CAD build for the part. Positions are in the model's coordinates, mm. A direction names the side the tool comes from. Round coordinates to 2 decimals unless told otherwise and drop trailing zeros. Loops run counter-clockwise (first coordinate to the right, second up) from the corner with the lowest first, then second, coordinate; pieces in that order, holes last. Notation, with made-up numbers: M 32,-32.5 L 50,-32.5 A10 ccw 50,-27.5 Z; hole C 14,71.25 d2. An arc over 180 degrees is marked long. Use one line per item in the form item = value.
Autodesk Inventor part; units mm, degrees
ref_plane "YZ Plane" through (0, 0, 0) normal (1, 0, 0) x (0, 1, 0)
ref_plane "XZ Plane" through (0, 0, 0) normal (0, 1, 0) x (-1, 0, 0)
ref_plane "XY Plane" through (0, 0, 0) normal (0, 0, 1) x (1, 0, 0)
sketch "スケッチ1" plane through (0, 0, 0) normal (0, 0, 1) x (1, 0, 0)
  line L0 (-17.5, 11) -> (17.5, 11)
  line L1 (17.5, 11) -> (17.5, -11)
  line L2 (17.5, -11) -> (-17.5, -11)
  line L3 (-17.5, -11) -> (-17.5, 11)
  point P0 (0, 0)
  point P1 (-17.5, 0)
  point P2 (0, 11)
  dimension "d0" = 35
  dimension "d1" = 22
extrude "押し出し1" add sketch "スケッチ1" along normal blind 1.6
sketch "スケッチ2" plane through (0, 0, 0) normal (0, 0, -1) x (-1, 0, 0)
  line L0 (15.24, 13.4783) -> (15.24, -13.8825) construction
  line L1 (17.5, 11) -> (17.5, -11) construction
  line L2 (18.6717, -5.08) -> (13.4177, -5.08) construction
  line L3 (17.5, -11) -> (-17.5, -11) construction
  line L4 (13.97, -6.35) -> (16.51, -6.35)
  line L5 (16.51, -6.35) -> (16.51, 6.35)
  line L6 (16.51, 6.35) -> (13.97, 6.35)
  line L7 (13.97, 6.35) -> (13.97, -6.35)
  point P0 (0, 0)
  point P1 (15.24, -6.35)
  dimension "d4" = 2.26
  dimension "d5" = 5.92
  dimension "d6" = 2.54
  dimension "d7" = 1.27
  dimension "d8" = 12.7
extrude "押し出し2" add sketch "スケッチ2" along normal blind 11
sketch "スケッチ3" plane through (0, 0, 1.6) normal (0, 0, 1) x (1, 0, 0)
  line L0 (-13, 10) -> (17, 10)
  line L1 (17, 10) -> (17, -9.5)
  line L2 (17, -9.5) -> (-13, -9.5)
  line L3 (-13, -9.5) -> (-13, 10)
  line L4 (17.5, 11) -> (-17.5, 11)
  line L5 (17.5, -11) -> (17.5, 11)
  point P0 (0, 0)
  dimension "d11" = 30
  dimension "d12" = 19.5
  dimension "d13" = 1
  dimension "d14" = 0.5
extrude "押し出し3" add sketch "スケッチ3" along normal blind 2
properties part number "PCB-AE-AQM0802"
1. Probe line 1 along Y through (x, z) = (1.5, 3.25); line 2 along Z through (x, y) = (-1.5, -3.75); line 3 along X through (y, z) = (-4, 2.75). List the from-to ranges inside material, lowest first. Write a range as from..to.
Completed:
line_1 = -9.5..10
line_2 = 0..3.6
line_3 = -13..17
2. Drop flat-ended pins along their axis: P1, Ø3, axis at x = -15.5, z = -6.5, coming from the +Y side; P2, Ø5, axis at y = 8, z = -4, coming from the -X side; P3, Ø1, axis at x = -2, z = 3, coming from the -Y side. Give the stop position or say it passes through.
Completed:
P1 = 6.35
P2 = -16.51
P3 = -9.5
3. Cut at C-C on z = -6.75. Write the cut outline in (x, y).
Completed:
outline = M -16.51,-6.35 L -13.97,-6.35 L -13.97,6.35 L -16.51,6.35 Z
4. Cut at A-A on y = -8. Write the cut outline in (x, z).
Completed:
outline = M -17.5,0 L 17.5,0 L 17.5,1.6 L 17,1.6 L 17,3.6 L -13,3.6 L -13,1.6 L -17.5,1.6 Z
5. Tool access for faces 1 (the face through (-15, -6.35, -5)), 2 (the face through (2, 10, 3)), 3 (the face through (-13.97, 0, -5)): list every direction of +Z, -Z, +X, -X, +Y, -Y with a clear straight run to the whole face (end or side of a thin tool).
Completed:
face_1 = -Z, +X, -X, -Y
face_2 = +Z, +X, -X, +Y
face_3 = -Z, +X, +Y, -Y
6. Cut at B-B on x = -9. Write the cut outline in (y, z), and give its area (3 significant figures).
Completed:
outline = M -11,0 L 11,0 L 11,1.6 L 10,1.6 L 10,3.6 L -9.5,3.6 L -9.5,1.6 L -11,1.6 Z
area = 74.2 mm2
7. Cut at D-D on y = -1. Write the cut outline in (x, z), and give its area (3 significant figures).
Completed:
outline = M -17.5,0 L -16.51,0 L -16.51,-11 L -13.97,-11 L -13.97,0 L 17.5,0 L 17.5,1.6 L 17,1.6 L 17,3.6 L -13,3.6 L -13,1.6 L -17.5,1.6 Z
area = 144 mm2
